Read the model definition and answer for the solid it produces. Units are mm, in the model's axes. A direction names the side the tool comes from. Coordinates: 2 decimals unless noted, no trailing zeros. Loops run counter-clockwise (first coordinate to the right, second up) from the corner with the lowest first, then second, coordinate; pieces in that order, holes last.
Q1. Section B-B (y = -181.5) is taken. Give the vertices of the cut face in (x, z).
Q2. Section A-A (z = -4.5) is taken. Give the vertices of the cut face in (x, y).
Q3. Flat-ended cylindrical pins translate along their axes: P1, Ø8, axis at x = 35, y = 66.75, coming from the -Z side; P2, Ø6, axis at y = -859, z = -11, coming from the -X side; P3, Ø6, axis at x = -8.5, z = -17, coming from the +Y side; P4, Ø4.5, axis at x = -35, y = 66.75, coming from the -Z side. Find the tip coordinate at first contact, or state that the pin passes through.
Q4. Straight lines are drawn through the part: line 1 (Y direction, x = -35, z = 2); line 2 (Y direction, x = 0, z = -12.25); line 3 (X direction, y = -364, z = -4). For each, find the intervals that lie inside material, in ascending order.
Q5. Which of the six approach directions +Z, -Z, +X, -X, +Y, -Y give full straight-line access (tool end or side, diameter ignored) to faces 1 (the face through (1, 1, 3)), 2 (the face through (0, -824, 0))?
from build123d import *

# Parameters (mm, degrees)
CROQUIS1_R                 = 2.5
SALIENTE_EXTRUIR1_DEPTH    = 3
SALIENTE_EXTRUIR2_DEPTH    = 20
CORTAR_EXTRUIR1_DEPTH      = 99
CORTAR_EXTRUIR1_DEPTH_BACK = 71
CROQUIS3_R                 = 2.5


with BuildPart() as part:
    # Croquis1 → Saliente-Extruir1 (new body)
    with BuildSketch(Plane.XY):
        with BuildLine():
            Line((-50, 85), (50, 85))
            ThreePointArc((50, 85), (71.213203436, 76.213203436), (80, 55))
            Line((80, 55), (80, -55))
            ThreePointArc((80, -55), (71.213203436, -76.213203436), (50, -85))
            Line((50, -85), (-50, -85))
            ThreePointArc((-50, -85), (-71.213203436, -76.213203436), (-80, -55))
            Line((-80, -55), (-80, 55))
            ThreePointArc((-80, 55), (-71.213203436, 76.213203436), (-50, 85))
        make_face()
        with Locations((0, -66.75)):
            Circle(CROQUIS1_R, mode=Mode.SUBTRACT)
        with Locations((0, 66.75)):
            Circle(CROQUIS1_R, mode=Mode.SUBTRACT)
        with Locations((-35, 66.75)):
            Circle(CROQUIS1_R, mode=Mode.SUBTRACT)
        with Locations((35, 66.75)):
            Circle(CROQUIS1_R, mode=Mode.SUBTRACT)
        with Locations((-35, -66.75)):
            Circle(CROQUIS1_R, mode=Mode.SUBTRACT)
        with Locations((35, -66.75)):
            Circle(CROQUIS1_R, mode=Mode.SUBTRACT)
    extrude(amount=SALIENTE_EXTRUIR1_DEPTH)

    # Croquis2 → Saliente-Extruir2 (add)
    with BuildSketch(Plane.XY):
        Polygon((-20, 0), (20, 0), (20, -665), (20, -1584.514762196), (-20, -1584.514762196), (-20, -665), align=None)
    extrude(amount=-SALIENTE_EXTRUIR2_DEPTH)

    # Croquis3 → Cortar-Extruir1 (cut, two sides: drawn at the far end of the back side and taken through both)
    with BuildSketch(Plane.XY.offset(-CORTAR_EXTRUIR1_DEPTH_BACK)):
        with Locations((0, -66.75)):
            Circle(CROQUIS3_R)
    extrude(amount=CORTAR_EXTRUIR1_DEPTH + CORTAR_EXTRUIR1_DEPTH_BACK, mode=Mode.SUBTRACT)


solid = part.part
Numbers:
1. outline: (-20, -20) - (20, -20) - (20, 0) - (-20, 0) - close
2. outline: (-20, -1584.51) - (20, -1584.51) - (20, 0) - (-20, 0) - close; hole circle Ø5 at (0, -66.75)
3. P1: stops at z = 0
3. P2: stops at x = -20
3. P3: stops at y = 0
3. P4: passes through
4. line 1: y = -85 to -69.25, -64.25 to 64.25, 69.25 to 85
4. line 2: y = -1584.51 to -69.25, -64.25 to 0
4. line 3: x = -20 to 20
5. face 1: +Z, +X, -X, +Y, -Y
5. face 2: +Z, +X, -X, -Y
